Read the model definition and answer for the solid it produces. Units are mm, in the model's axes. A direction names the side the tool comes from. Give positions to 0.01 mm unless a question says otherwise; leave off trailing zeros. Order: outer loops, then holes, each group sorted by start corner. A loop starts at its lowest first (then second) coordinate and runs counter-clockwise, first axis right, second up. Notation, with made-up numbers: M 6.25,62.5 L 36.25,62.5 A26 ccw 36.25,92.5 Z; hole C -22.5,-5.5 d4. An arc over 180 degrees is marked long. One line per item, written item: value. Start each with the question number.
from build123d import *

# Parameters (mm, degrees)
SKETCH1_R           = 3.429
SKETCH1_R_2         = 2.54
BOSS_EXTRUDE1_DEPTH = 3.2004
SKETCH2_R           = 2.413
CUT_EXTRUDE1_DEPTH  = 3.2004
SKETCH3_R           = 2.159
CUT_EXTRUDE2_DEPTH  = 3.2004
SKETCH6_W           = 107.95
SKETCH6_H           = 3.2512
CUT_EXTRUDE3_DEPTH  = 3.2004
SKETCH7_R           = 3.429
CUT_EXTRUDE4_DEPTH  = 3.2004
CUT_EXTRUDE5_DEPTH  = 3.2004
CUT_EXTRUDE6_DEPTH  = 3.2004
BOSS_EXTRUDE2_DEPTH = 3.2004
SKETCH13_R          = 1.1303
CUT_EXTRUDE7_DEPTH  = 3.2004
CUT_EXTRUDE8_DEPTH  = 3.2004
FILLET1_R           = 5.08
SKETCH16_R          = 1.1303
SKETCH16_R_2        = 1.025
CUT_EXTRUDE9_DEPTH  = 3.2004
SKETCH20_R          = 2.159
CUT_EXTRUDE11_DEPTH = 3.2004


with BuildPart() as part:
    # Sketch1 → Boss-Extrude1 (new body)
    with BuildSketch(Plane.XY):
        with BuildLine():
            Line((0, 0), (120.015, 0))
            ThreePointArc((120.015, 0), (130.351788396, 3.075697789), (137.325636158, 11.302152592))
            Line((137.325636158, 11.302152592), (155.2575, 52.11572))
            ThreePointArc((155.2575, 52.11572), (157.54731739, 67.602183396), (151.630955452, 82.09599151))
            ThreePointArc((151.630955452, 82.09599151), (60.0075, 127.266502568), (-31.615955452, 82.09599151))
            ThreePointArc((-31.615955452, 82.09599151), (-37.53231739, 67.602183396), (-35.2425, 52.11572))
            Line((-35.2425, 52.11572), (-17.310636158, 11.302152592))
            ThreePointArc((-17.310636158, 11.302152592), (-10.336788396, 3.075697789), (0, 0))
        make_face()
        with Locations((120.015, 18.90776)):
            Circle(SKETCH1_R, mode=Mode.SUBTRACT)
        with Locations((0, 18.90776)):
            Circle(SKETCH1_R_2, mode=Mode.SUBTRACT)
        with Locations((19.734727626, 25.566426992)):
            Circle(SKETCH1_R_2, mode=Mode.SUBTRACT)
    extrude(amount=BOSS_EXTRUDE1_DEPTH)

    # Sketch2 → Cut-Extrude1 (cut)
    with BuildSketch(Plane(origin=(0, 0, 0), x_dir=(-1, 0, 0), z_dir=(0, 0, -1))):
        with Locations((-92.0115, 52.11572)):
            Circle(SKETCH2_R)
        with Locations((-76.0095, 52.11572)):
            Circle(SKETCH2_R)
        with Locations((-44.0055, 52.11572)):
            Circle(SKETCH2_R)
        with Locations((-28.0035, 52.11572)):
            Circle(SKETCH2_R)
    extrude(amount=-CUT_EXTRUDE1_DEPTH, mode=Mode.SUBTRACT)

    # Sketch3 → Cut-Extrude2 (cut)
    with BuildSketch(Plane.XY.offset(3.2004)):
        with Locations((21.9075, 3.81)):
            Circle(SKETCH3_R)
        with Locations((60.0075, 3.81)):
            Circle(SKETCH3_R)
        with Locations((98.1075, 3.81)):
            Circle(SKETCH3_R)
    extrude(amount=-CUT_EXTRUDE2_DEPTH, mode=Mode.SUBTRACT)

    # Sketch6 → Cut-Extrude3 (cut)
    with BuildSketch(Plane(origin=(0, 0, 0), x_dir=(-1, 0, 0), z_dir=(0, 0, -1))):
        with Locations((-60.0075, 46.68012)):
            Rectangle(SKETCH6_W, SKETCH6_H)
    extrude(amount=-CUT_EXTRUDE3_DEPTH, mode=Mode.SUBTRACT)

    # Sketch7 → Cut-Extrude4 (cut)
    with BuildSketch(Plane.XY.offset(3.2004)):
        with Locations((126.474462556, 80.535782848)):
            Circle(SKETCH7_R)
    extrude(amount=-CUT_EXTRUDE4_DEPTH, mode=Mode.SUBTRACT)

    # Sketch11 → Cut-Extrude5 (cut)
    with BuildSketch(Plane.XY.offset(3.2004)):
        with BuildLine():
            Line((121.0824837, 109.799267349), (93.538394554, 93.734155779))
            Line((93.538394554, 93.734155779), (34.363029741, 105.455155066))
            Line((34.363029741, 105.455155066), (38.27464621, 125.20358486))
            ThreePointArc((38.27464621, 125.20358486), (81.132699311, 125.318307405), (121.0824837, 109.799267349))
        make_face()
    extrude(amount=-CUT_EXTRUDE5_DEPTH, mode=Mode.SUBTRACT)

    # Sketch12 → Cut-Extrude6 (cut)
    with BuildSketch(Plane.XY.offset(3.2004)):
        with BuildLine():
            Line((35.641093634, 114.854322507), (36.202710537, 114.743081768))
            Line((36.202710537, 114.743081768), (38.27464621, 125.20358486))
            ThreePointArc((38.27464621, 125.20358486), (32.033357942, 123.827921759), (25.877709031, 122.109167938))
            ThreePointArc((25.877709031, 122.109167938), (29.941556488, 117.381110641), (35.641093634, 114.854322507))
        make_face()
    extrude(amount=-CUT_EXTRUDE6_DEPTH, mode=Mode.SUBTRACT)

    # Sketch14 → Boss-Extrude2 (add)
    with BuildSketch(Plane.XY.offset(3.2004)):
        with BuildLine():
            Line((-44.811597123, 54.685748683), (-19.142507527, 10.95973357))
            ThreePointArc((-19.142507527, 10.95973357), (-11.028954555, 2.933815076), (0, 0))
            ThreePointArc((0, 0), (-12.648210364, 66.477064779), (25.877709031, 122.109167938))
            ThreePointArc((25.877709031, 122.109167938), (-10.925402455, 107.037965152), (-41.85988351, 82.044605027))
            ThreePointArc((-41.85988351, 82.044605027), (-47.856144624, 68.852877757), (-44.811597123, 54.685748683))
        make_face()
    extrude(amount=-BOSS_EXTRUDE2_DEPTH)

    # Sketch13 → Cut-Extrude7 (cut)
    with BuildSketch(Plane.XY.offset(3.2004)):
        with Locations((44.1325, 81.07172)):
            Circle(SKETCH13_R)
        with Locations((44.1325, 60.75172)):
            Circle(SKETCH13_R)
        with Locations((18.7325, 60.75172)):
            Circle(SKETCH13_R)
        with Locations((18.7325, 81.07172)):
            Circle(SKETCH13_R)
        with Locations((6.0325, 81.07172)):
            Circle(SKETCH13_R)
        with Locations((6.0325, 60.75172)):
            Circle(SKETCH13_R)
        with Locations((-19.3675, 60.75172)):
            Circle(SKETCH13_R)
        with Locations((-19.3675, 81.07172)):
            Circle(SKETCH13_R)
    extrude(amount=-CUT_EXTRUDE7_DEPTH, mode=Mode.SUBTRACT)

    # Sketch15 → Cut-Extrude8 (cut)
    with BuildSketch(Plane.XY.offset(3.2004)):
        with BuildLine():
            Line((79.0575, 73.70572), (104.4575, 73.70572))
            ThreePointArc((104.4575, 73.70572), (110.8075, 67.35572), (104.4575, 61.00572))
            Line((104.4575, 61.00572), (79.0575, 61.00572))
            ThreePointArc((79.0575, 61.00572), (72.7075, 67.35572), (79.0575, 73.70572))
        make_face()
        with BuildLine():
            Line((78.4225, 22.08276), (97.4725, 22.08276))
            ThreePointArc((97.4725, 22.08276), (100.6475, 18.90776), (97.4725, 15.73276))
            Line((97.4725, 15.73276), (78.4225, 15.73276))
            ThreePointArc((78.4225, 15.73276), (75.2475, 18.90776), (78.4225, 22.08276))
        make_face()
    extrude(amount=-CUT_EXTRUDE8_DEPTH, mode=Mode.SUBTRACT)

    # Fillet1
    fillet1_edges = [part.edges().sort_by_distance(p)[0] for p in [
        (121.0824837, 109.799267349, 1.6002),
        (36.202710537, 114.743081768, 1.6002),
        (25.877709031, 122.109167938, 1.6002),
    ]]
    fillet(fillet1_edges, radius=FILLET1_R)

    # Sketch16 → Cut-Extrude9 (cut)
    with BuildSketch(Plane.XY.offset(3.2004)):
        with Locations((112.438115095, 24.679799513)):
            Circle(SKETCH16_R)
        with Locations((127.591884905, 13.135720487)):
            Circle(SKETCH16_R)
        with Locations((120.029328249, 76.814682821)):
            Circle(SKETCH16_R_2)
        with Locations((132.919596863, 84.256882875)):
            Circle(SKETCH16_R_2)
    extrude(amount=-CUT_EXTRUDE9_DEPTH, mode=Mode.SUBTRACT)

    # Sketch20 → Cut-Extrude11 (cut)
    with BuildSketch(Plane.XY.offset(3.2004)):
        with Locations((8.255, 18.90776)):
            Circle(SKETCH20_R)
        with Locations((109.47654, 18.90776)):
            Circle(SKETCH20_R)
    extrude(amount=-CUT_EXTRUDE11_DEPTH, mode=Mode.SUBTRACT)


solid = part.part
Q1. Find section C-C, the plane x = -6.5. Give the vertices of the cut face in (y, z).
Q2. Determine the mould class of faces 1 (the flat face through (53, 62, 0)), 2 (the cylindrical face through (-47.833, 69.058, 1.623)), 3 (the cylindrical face through (20.19, 2.5, 1.62)), 4 (the cylindrical face through (-12.025, 106.381, 1.623)) for opening direction Y: released by +Y, released by -Y, zero draft, split by the parting line, or undercut.
Q3. Find section B-B, the plane z = 2.4. State how many separate pieces and enclosed holes the cut face has, then the cut area to 3 significant figures.
Q4. Consider probe 1 along Y at (x, z) = (6, 1.6); probe 2 along Y at (x, z) = (19.5, 0.75); probe 3 along Y at (x, z) = (119.5, 1.4). Determine where each line is inside the solid, lowest interval first.
Q5. Each of these flat-tipped pins is pushed along its axis until it touches: pin 1 (1 mm diameter, centred on x = 93.5, z = 1.5, fed in from +Y); pin 2 (1.6 mm diameter, centred on x = 86.5, z = 2, fed in from +Y); pin 3 (1 mm diameter, centred on y = 55, z = 2.5, fed in from -X). Where does it stop, or does it pass through?
Q6. Find section A-A, the plane y = 3.81. Give the vertices of the cut face in (x, z).
Q7. A tool of negligible diameter and unlimited length cuts with its end or side. For faces 5 (the flat face through (106.141, 101.085, 1.623)), 6 (the cylindrical face through (29.792, 117.494, 1.623)), 7 (the cylindrical face through (72.71, 67.22, 1.62)), from which of +Z, -Z, +X, -X, +Y, -Y can it reach the whole face along a straight path? Write none if from no direction.
Evaluation:
1. outline: M 0.97,0 L 109.55,0 L 109.55,3.2 L 0.97,3.2 Z
2. face 1: zero draft
2. face 2: split by the parting line
2. face 3: undercut
2. face 4: released by +Y
3. separate pieces: 1
3. enclosed holes: 28
3. area: 17,700 mm2
4. probe 1: 0 to 59.62, 61.88 to 79.94, 82.2 to 115.53
4. probe 2: 0 to 23.04, 28.1 to 45.05, 48.31 to 59.92, 61.58 to 80.24, 81.9 to 120.36
4. probe 3: 0 to 15.52, 22.3 to 75.94, 77.69 to 108.71
5. pin 1: y = 94
5. pin 2: y = 95.29
5. pin 3: x = -45.27
6. outline: M -12.43,0 L 19.75,0 L 19.75,3.2 L -12.43,3.2 Z; M 24.07,0 L 57.85,0 L 57.85,3.2 L 24.07,3.2 Z; M 62.17,0 L 95.95,0 L 95.95,3.2 L 62.17,3.2 Z; M 100.27,0 L 131.4,0 L 131.4,3.2 L 100.27,3.2 Z
7. face 5: +Z, -Z, +Y
7. face 6: +Z, -Z, +X, +Y
7. face 7: +Z, -Z
